Could you check a few things on this drawing? It's one solid part, dimensions in mm from its lowest x, y, z. Give positions to 0.01 mm unless a question says otherwise; leave off trailing zeros. Loops run counter-clockwise (first coordinate to the right, second up) from the corner with the lowest first, then second, coordinate; pieces in that order, holes last. Notation, with made-up numbers: (61.5, -31.5) - (93.5, -31.5) arc R29 cw to (93.5, -0.5) - close; hole circle Ø1 at (59.25, 36). An arc over 180 degrees is marked (long way). Write each question's results on one line, items separated by ' | '. Start each with the question number.
(1) Suppose I cut it at C-C (y = 31). Please give me the cut outline in (x, z).
(2) Suppose I cut it at A-A (z = 45). Please give me the cut outline in (x, y) (1 decimal), and give its area (3 significant figures).
(3) For pin 1 (2 mm diameter, centred on x = 75, z = 75, fed in from -Y); pin 2 (1 mm diameter, centred on x = 42, y = 332.5, fed in from -Z); pin 3 (4 mm diameter, centred on y = 69, z = 42, fed in from -X); pin 4 (22 mm diameter, centred on x = 45, z = 45, fed in from +Y), each with a flat end and sliding along its axis, tell me the tip position at first contact or that it passes through.
(4) If we mould it in two halves opening along Z, with no side actions, what happens to the marked faces 1, 2 and 3? For each: released by +Z, released by -Z, zero draft, split by the parting line, or undercut.
(5) Suppose I cut it at B-B (x = 45). Please give me the cut outline in (y, z) (1 decimal), and give its area (3 significant figures).
(6) I need wall thicknesses on line 1 (X direction, y = 291, z = 45); line 2 (Z direction, x = 34, y = 306) (1 decimal); line 3 (X direction, y = 241, z = 52). Which ranges of each line are inside material? Lowest first, please.
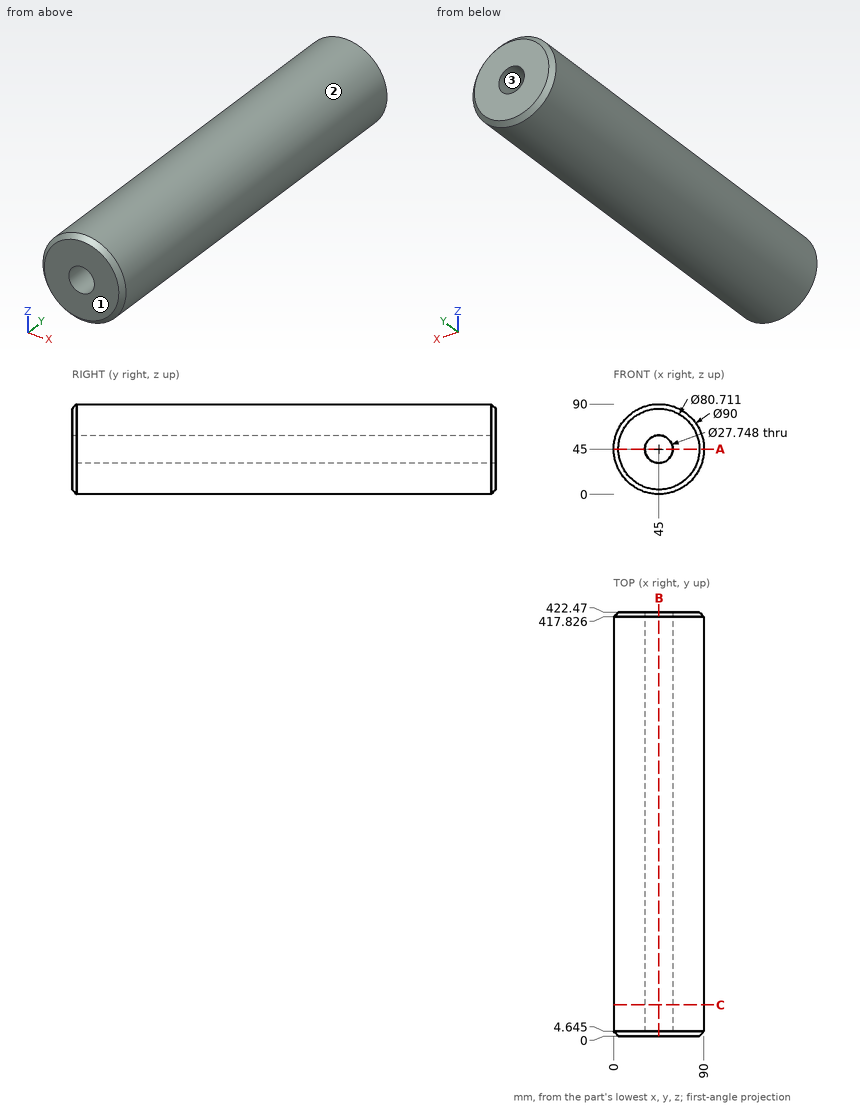
Output values:
1) outline: circle Ø90 at (45, 45); hole circle Ø27.75 at (45, 45)
2) outline: (0, 4.6) - (4.6, 0) - (31.1, 0) - (31.1, 422.5) - (4.6, 422.5) - (0, 417.8) - close; (58.9, 0) - (85.4, 0) - (90, 4.6) - (90, 417.8) - (85.4, 422.5) - (58.9, 422.5) - close | area: 26,300 mm2
3) pin 1: y = 1.07 | pin 2: z = 0.07 | pin 3: x = 0.01 | pin 4: through
4) face 1: zero draft | face 2: split by the parting line | face 3: undercut
5) outline: (0, 4.6) - (4.6, 0) - (417.8, 0) - (422.5, 4.6) - (422.5, 31.1) - (0, 31.1) - close; (0, 58.9) - (422.5, 58.9) - (422.5, 85.4) - (417.8, 90) - (4.6, 90) - (0, 85.4) - close | area: 26,300 mm2
6) line 1: 0 to 31.13, 58.87 to 90 | line 2: 1.4 to 36.5, 53.5 to 88.6 | line 3: 0.55 to 33.02, 56.98 to 89.45
